Input: part model. Units: mm. Frame: model coordinates. A direction names the side the tool comes from. Coordinates: 2 decimals unless noted, no trailing zeros. Write each loop counter-clockwise with the first axis right and the second up, starting at its lowest first coordinate (ties: lowest second). Pieces come first, ordered by that corner, then holes. Notation, with made-up numbers: M -17.75,-37.75 L 29.25,-37.75 A14 ccw 29.25,-31.75 Z; hole C -30,21.25 d7. An arc over 180 degrees is marked long. Answer as a JSON object with one key per item and string values. Group by question number.
from build123d import *

# Parameters (mm, degrees)
F0_W     = 100
F0_H     = 50
F1_DEPTH = 15
F2_W     = 15
F2_H     = 50
F3_DEPTH = 85
F4_W     = 30
F4_H     = 10.7893505692
F4_H_2   = 10
F5_DEPTH = 30
F6_SIZE  = 29.99999
F7_R     = 12.5
F8_R     = 12.5
F9_DEPTH = 25
F10_R    = 24.99999
F11_SIZE = 1


# Not quite as in the source:
# - a fillet or chamfer is up to 0.001 mm smaller than in the source, because OpenCascade refuses the exact size


with BuildPart() as f1:
    # F0 (on Top) → F1 (new body)
    with BuildSketch(Plane.XY):
        with Locations((1.2109465897, -8.8487002536)):
            Rectangle(F0_W, F0_H)
    extrude(amount=F1_DEPTH)

    # F2 (on face) → F3 (join)
    with BuildSketch(Plane.XY.offset(15)):
        with Locations((-41.2890534103, -8.8487002536)):
            Rectangle(F2_W, F2_H)
    extrude(amount=F3_DEPTH)

    # F4 (on face) → F5 (join)
    with BuildSketch(Plane.XY.offset(15)):
        with Locations((-18.7890534103, -28.454024969)):
            Rectangle(F4_W, F4_H)
        with Locations((-18.7890534103, 11.1512997464)):
            Rectangle(F4_W, F4_H_2)
    extrude(amount=F5_DEPTH)

    # F6 (size 30 in the source; OpenCascade refuses exactly that, so slightly less here)
    f6_edges = [f1.edges().sort_by_distance(p)[0] for p in [
        (-3.789053, 11.1513, 45),
        (-3.789053, -28.454025, 45),
    ]]
    chamfer(f6_edges, length=F6_SIZE)

    # F7 (on face) + F8 (on face) → F9 (cut)
    with BuildSketch(Plane(origin=(-48.7890534103, 0, 0), x_dir=(0, -1, 0), z_dir=(-1, 0, 0))):
        with Locations((8.8487002536, 75)):
            Circle(F7_R)
    with BuildSketch(Plane(origin=(-48.7890534103, 0, 0), x_dir=(0, -1, 0), z_dir=(-1, 0, 0))):
        with Locations((8.8487002536, 75)):
            Circle(F8_R)
    extrude(amount=-F9_DEPTH, mode=Mode.SUBTRACT)

    # F10 (radius 25 in the source; OpenCascade refuses exactly that, so slightly less here)
    f10_edges = [f1.edges().sort_by_distance(p)[0] for p in [
        (-41.289053, 16.1513, 100),
        (-41.289053, -33.8487, 100),
    ]]
    fillet(f10_edges, radius=F10_R)

    # F11
    f11_edges = [f1.edges().sort_by_distance(p)[0] for p in [
        (-33.789053, 3.6513, 75),
        (-48.789053, 3.6513, 75),
    ]]
    chamfer(f11_edges, length=F11_SIZE)


solid = f1.part
Q1. Section C-C, the plane x = -15. Return the cut outline in (y, z), and give its area (3 significant figures).
Q2. Section A-A, the plane z = 28.5. Return the cut outline in (x, y).
Q3. Pin query (flat end, axial travel): pin 1 Ø25 at (y, z) = (-16, 78.5) entering from +X; pin 2 Ø15 at (y, z) = (-8.85, 75) entering from +X. Return the tip coordinate at first contact, or that it passes through.
Q4. Section D-D, the plane z = 55.5. Return the cut outline in (x, y), and give its area (3 significant figures).
Q5. Access query for faces 1 (the cylindrical face through (-41.184, 8.634, 92.871)), 2 (the flat face through (-22, 6.151, 26)). Directions: +Z, -Z, +X, -X, +Y, -Y. A direction counts if a zero-diameter tool reaches every point of the face in a straight line with its end or side. Return the directions, or none.
Q6. Draft query along Y for faces 3 (the flat face through (-22, -23.059, 26)), 4 (the flat face through (-18.58, 11.08, 29.79)), 5 (the cylindrical face through (-41.2, -26.7, 92.5)), 6 (the flat face through (-11, 16.151, 20)). Return one class per face: released by +Y, released by -Y, zero draft, split by the parting line, or undercut.
Q7. Line query: line 1 (X direction, y = -18, z = 58); line 2 (Z direction, x = 14, y = -2); line 3 (Y direction, x = -41, z = 81). Output: solid intervals per line, ascending. Write a range as from..to.
Filled in:
{
 "1": {"outline": "M -33.85,0 L 16.15,0 L 16.15,26.21 L 6.15,26.21 L 6.15,15 L -23.06,15 L -23.06,26.21 L -33.85,26.21 Z", "area": "983 mm^2"},
 "2": {"outline": "M -48.79,-33.85 L -17.29,-33.85 L -17.29,-23.06 L -33.79,-23.06 L -33.79,6.15 L -17.29,6.15 L -17.29,16.15 L -48.79,16.15 Z"},
 "3": {"pin 1": "x = -33.79", "pin 2": "through"},
 "4": {"outline": "M -48.79,-33.85 L -33.79,-33.85 L -33.79,16.15 L -48.79,16.15 Z", "area": "750 mm^2"},
 "5": {"face 1": "+Z, +X, -X, +Y", "face 2": "+Z, +X"},
 "6": {"face 3": "undercut", "face 4": "zero draft", "face 5": "released by -Y", "face 6": "released by +Y"},
 "7": {"line 1": "-48.79..-33.79", "line 2": "0..15", "line 3": "-33.12..-19.81, 2.12..15.42"}
}
